Could you check a few things on this model? Use its own coordinates, in mm. Coordinates: 2 decimals unless noted, no trailing zeros. Write each loop counter-clockwise with the first axis right and the second up, starting at its lowest first coordinate (ties: lowest second). Pieces come first, ordered by that corner, then holes.
```python
from build123d import *

# Parameters (mm, degrees)
SKETCH_W        = 113.3828
SKETCH_H        = 73.3828
SKETCH_R        = 8.784219
PAD_DEPTH       = 10
CHAMFER_SIZE    = 1
CHAMFER001_SIZE = 1
CHAMFER002_SIZE = 1
CHAMFER003_SIZE = 1


with BuildPart() as part:
    # Sketch → Pad (new body)
    with BuildSketch(Plane.XY):
        Rectangle(SKETCH_W, SKETCH_H)
        with Locations((-40, 20)):
            Circle(SKETCH_R, mode=Mode.SUBTRACT)
        with Locations((-40, -20)):
            Circle(SKETCH_R, mode=Mode.SUBTRACT)
        with Locations((40, -20)):
            Circle(SKETCH_R, mode=Mode.SUBTRACT)
        with Locations((40, 20)):
            Circle(SKETCH_R, mode=Mode.SUBTRACT)
    extrude(amount=PAD_DEPTH)

    # Chamfer
    chamfer_edges = [part.edges().sort_by_distance(p)[0] for p in [
        (31.215781, 20, 10),
    ]]
    chamfer(chamfer_edges, length=CHAMFER_SIZE)

    # Chamfer001
    chamfer001_edges = [part.edges().sort_by_distance(p)[0] for p in [
        (31.215781, -20, 10),
    ]]
    chamfer(chamfer001_edges, length=CHAMFER001_SIZE)

    # Chamfer002
    chamfer002_edges = [part.edges().sort_by_distance(p)[0] for p in [
        (-48.784219, 20, 10),
    ]]
    chamfer(chamfer002_edges, length=CHAMFER002_SIZE)

    # Chamfer003
    chamfer003_edges = [part.edges().sort_by_distance(p)[0] for p in [
        (-48.784219, -20, 10),
    ]]
    chamfer(chamfer003_edges, length=CHAMFER003_SIZE)


solid = part.part
```
Item 1: I want a section at C-C, the plane x = 40. List the corners of the cut face in (y, z) for me, then the cut area to 3 significant figures.
Item 2: I want a section at A-A, the plane y = -20. List the corners of the cut face in (x, z) for me.
Item 3: If we mould it in two halves opening along X, with no side actions, what happens to faces 1 (the flat face through (-56.691, -1, 5)), 2 (the cylindrical face through (-31.9, 16.6, 4.4)), 3 (the flat face through (-1, 1, 0))? For each: released by +X, released by -X, zero draft, split by the parting line, or undercut.
Item 4: I want a section at B-B, the plane z = 7.25. List the corners of the cut face in (x, y) for me.
Item 5: If I drill on line 1 along Y through (x, z) = (40, 4); line 2 along Y through (x, z) = (45.5, 9.25); line 3 along X through (y, z) = (-23, 6), over which ranges is the centre line in solid material (lowest first)?
Taken from the geometry:
1. outline: (-36.69, 0) - (-28.78, 0) - (-28.78, 9) - (-29.78, 10) - (-36.69, 10) - close; (-11.22, 0) - (11.22, 0) - (11.22, 9) - (10.22, 10) - (-10.22, 10) - (-11.22, 9) - close; (28.78, 0) - (36.69, 0) - (36.69, 10) - (29.78, 10) - (28.78, 9) - close
1. area: 380 mm2
2. outline: (-56.69, 0) - (-48.78, 0) - (-48.78, 9) - (-49.78, 10) - (-56.69, 10) - close; (-31.22, 0) - (31.22, 0) - (31.22, 9) - (30.22, 10) - (-30.22, 10) - (-31.22, 9) - close; (48.78, 0) - (56.69, 0) - (56.69, 10) - (49.78, 10) - (48.78, 9) - close
3. face 1: released by -X
3. face 2: undercut
3. face 3: zero draft
4. outline: (-56.69, -36.69) - (56.69, -36.69) - (56.69, 36.69) - (-56.69, 36.69) - close; hole circle Ø17.57 at (-40, -20); hole circle Ø17.57 at (-40, 20); hole circle Ø17.57 at (40, -20); hole circle Ø17.57 at (40, 20)
5. line 1: y = -36.69 to -28.78, -11.22 to 11.22, 28.78 to 36.69
5. line 2: y = -36.69 to -27.17, -12.83 to 12.83, 27.17 to 36.69
5. line 3: x = -56.69 to -48.26, -31.74 to 31.74, 48.26 to 56.69
